Geometry: see drawing. Coordinates: mm, zero at the bounding-box minimum. A direction names the side the tool comes from. Give positions to 0.01 mm unless a question says otherwise; leave off trailing zeros. Write each loop counter-clockwise with the first axis right and the second up, starting at its lowest first coordinate (ties: lowest second). Pieces come first, ordered by that corner, then holes. Notation, with made-up numbers: M -14,77.25 L 29,77.25 A27 cw 29,106.25 Z; hole C 2,39 d2. An arc over 180 degrees is marked long. Use a Markdown table: item, result. Add a question column.
1) Pin query (flat end, axial travel): pin 1 (2.5 mm diameter, centred on x = 23.18, y = 4.94, fed in from +Z) (1 decimal); pin 2 (1.2 mm diameter, centred on x = 7, y = 13, fed in from +Z); pin 3 (2 mm diameter, centred on x = 34, y = 35, fed in from -Z). Return the tip coordinate at first contact, or that it passes through.
2) Line query: line 1 (Y direction, x = 30, z = 2.75); line 2 (Y direction, x = 40.5, z = 6.5) (1 decimal); line 3 (X direction, y = 55, z = 3). Output: solid intervals per line, ascending.
3) Section B-B on x = 10. Return the cut outline in (y, z).
4) Draft query along X for the marked faces 1, 2 and 3. Return one class per face: +X half, -X half, draft (parallel to the pull), parting line (faces both ways), or undercut.
5) Section C-C on z = 8.75. State how many separate pieces and enclosed holes the cut face has, then the cut area to 3 significant figures.
6) Set-up query: the marked faces 4 and 5. Return all of +Z, -Z, +X, -X, +Y, -Y with unobstructed straight access to the full face (end or side cutting, diameter ignored); none if empty.
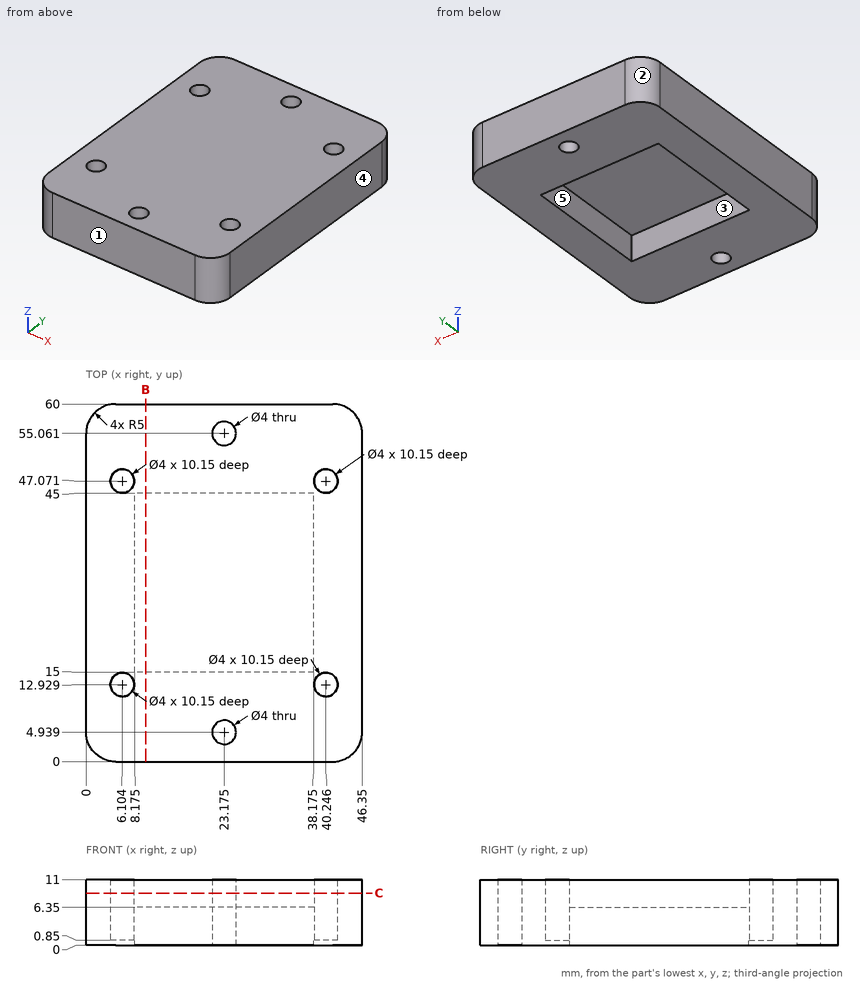
Found:
| question | item | result |
|---|---|---|
| 1 | pin 1 | through |
| 1 | pin 2 | z = 0.85 |
| 1 | pin 3 | z = 6.35 |
| 2 | line 1 | 0 to 15, 45 to 60 |
| 2 | line 2 | 0 to 10.9, 14.9 to 45.1, 49.1 to 60 |
| 2 | line 3 | 0 to 21.18, 25.17 to 46.35 |
| 3 | outline | M 0,0 L 15,0 L 15,6.35 L 45,6.35 L 45,0 L 60,0 L 60,11 L 0,11 Z |
| 4 | face 1 | draft |
| 4 | face 2 | -X half |
| 4 | face 3 | undercut |
| 5 | separate pieces | 1 |
| 5 | enclosed holes | 6 |
| 5 | area | 2,680 mm² |
| 6 | face 4 | +Z, -Z, +X, +Y, -Y |
| 6 | face 5 | -Z |
